Geometry: final body of the model. Coordinates: model frame, mm. A direction names the side the tool comes from. Coordinates: 2 decimals unless noted, no trailing zeros. Loops run counter-clockwise (first coordinate to the right, second up) from the corner with the lowest first, then second, coordinate; pieces in that order, holes last. Notation, with made-up numbers: (-28, 78.25) - (-2, 78.25) arc R11 cw to (-2, 85.25) - close; hole circle Ø5 at (69.25, -40). An arc over 180 degrees is marked (long way). Answer in a Markdown table with one row per item.
from build123d import *

# Parameters (mm, degrees)
SKETCH_1_R               = 23.5
EXTRUDE_1_DEPTH          = 4
SKETCH_2_R               = 5.85
EXTRUDE_2_DEPTH          = 7
SKETCH_3_R               = 2.5
CUT_EXTRUDE_1_DEPTH      = 3.4
SKETCH_4_R               = 2.1
CUT_EXTRUDE_2_DEPTH      = 5
PATTERN_CIRCULAR_1_COUNT = 4
SKETCH_5_R               = 2
CUT_EXTRUDE_3_DEPTH      = 8.6


with BuildPart() as part:
    # 草圖1 → 填料-伸長1 (new body)
    with BuildSketch(Plane(origin=(0, 0, 0), x_dir=(1, 0, 0), z_dir=(0, 1, 0))):
        Circle(SKETCH_1_R)
    extrude(amount=EXTRUDE_1_DEPTH)

    # 草圖2 → 填料-伸長2 (add)
    with BuildSketch(Plane(origin=(0, 4, 0), x_dir=(1, 0, 0), z_dir=(0, 1, 0))):
        Circle(SKETCH_2_R)
    extrude(amount=EXTRUDE_2_DEPTH)

    # 草圖3 → 除料-伸長1 (cut)
    with BuildSketch(Plane(origin=(0, 11, 0), x_dir=(1, 0, 0), z_dir=(0, 1, 0))):
        Circle(SKETCH_3_R)
    extrude(amount=-CUT_EXTRUDE_1_DEPTH, mode=Mode.SUBTRACT)

    # 草圖4 → 除料-伸長2 (cut, through all)
    with BuildSketch(Plane(origin=(0, 4, 0), x_dir=(1, 0, 0), z_dir=(0, 1, 0))):
        with Locations((-15.5, 0)):
            Circle(SKETCH_4_R)
        with Locations((-15.5, 8.5)):
            Circle(SKETCH_4_R)
        with Locations((-15.5, -8.5)):
            Circle(SKETCH_4_R)
    cut_extrude_2 = extrude(amount=-CUT_EXTRUDE_2_DEPTH, mode=Mode.SUBTRACT)

    # 環狀複製排列1: 除料-伸長2 ×4 about axis
    pattern_circular_1_axis = Axis((0, 0, 0), (0, 1, 0))
    for i in range(1, PATTERN_CIRCULAR_1_COUNT):
        add(cut_extrude_2.rotate(pattern_circular_1_axis, i * 360 / PATTERN_CIRCULAR_1_COUNT), mode=Mode.SUBTRACT)

    # 草圖5 → 除料-伸長3 (cut, through all)
    with BuildSketch(Plane(origin=(0, 7.6, 0), x_dir=(1, 0, 0), z_dir=(0, 1, 0))):
        Circle(SKETCH_5_R)
    extrude(amount=-CUT_EXTRUDE_3_DEPTH, mode=Mode.SUBTRACT)


solid = part.part
(1) First-contact query: pin 1 Ø5 at (x, z) = (-7.5, 10.5) entering from -Y; pin 2 Ø2 at (x, y) = (-1, 7.5) entering from +Z; pin 3 Ø5.5 at (x, z) = (-15.5, 0) entering from +Y; pin 4 Ø2.5 at (x, z) = (-1, -0.5) entering from +Y. Flat tips, straight axial feed; report the tip coordinate or a pass-through.
Verdict:
| item | result |
|---|---|
| pin 1 | stops at y = 0 |
| pin 2 | stops at z = 5.85 |
| pin 3 | stops at y = 4 |
| pin 4 | stops at y = 7.6 |
(2) Cut plane A-A on y = 1.75. State how many separate pieces and enclosed holes the cut face has, then the cut area to 3 significant figures.
Verdict:
| item | result |
|---|---|
| separate pieces | 1 |
| enclosed holes | 13 |
| area | 1,560 mm² |
(3) Cut plane B-B on z = -7. Output: boundary loops of the cut face in (x, y).
Verdict:
| item | result |
|---|---|
| outline | (-22.43, 0) - (-16.97, 0) - (-16.97, 4) - (-22.43, 4) - close; (-14.03, 0) - (14.03, 0) - (14.03, 4) - (-14.03, 4) - close; (16.97, 0) - (22.43, 0) - (22.43, 4) - (16.97, 4) - close |
(4) Access query for faces 4 (the face through (-1, 7.6, -2)), 5 (the face through (0, 0, 5)). Directions: +Z, -Z, +X, -X, +Y, -Y. A direction counts if a zero-diameter tool reaches every point of the face in a straight line with its end or side. Return the directions, or none.
Verdict:
| item | result |
|---|---|
| face 4 | +Y |
| face 5 | +Z, -Z, +X, -X, -Y |
(5) Ray query, probe 1 along X at (y, z) = (3.25, -15.5); probe 2 along Z at (x, y) = (0, 5.5); probe 3 along Z at (x, y) = (0, 9.55). Return the intervals inside material, ascending.
Verdict:
| item | result |
|---|---|
| probe 1 | x = -17.66 to -10.6, -6.4 to -2.1, 2.1 to 6.4, 10.6 to 17.66 |
| probe 2 | z = -5.85 to -2, 2 to 5.85 |
| probe 3 | z = -5.85 to -2.5, 2.5 to 5.85 |
(6) Cut plane D-D on z = 0. Output: boundary loops of the cut face in (x, y), then the cut area to 3 significant figures.
Verdict:
| item | result |
|---|---|
| outline | (-23.5, 0) - (-17.6, 0) - (-17.6, 4) - (-23.5, 4) - close; (-13.4, 0) - (-2, 0) - (-2, 7.6) - (-2.5, 7.6) - (-2.5, 11) - (-5.85, 11) - (-5.85, 4) - (-13.4, 4) - close; (2, 0) - (13.4, 0) - (13.4, 4) - (5.85, 4) - (5.85, 11) - (2.5, 11) - (2.5, 7.6) - (2, 7.6) - close; (17.6, 0) - (23.5, 0) - (23.5, 4) - (17.6, 4) - close |
| area | 189 mm² |
(7) Cut plane C-C on x = 10. Output: boundary loops of the cut face in (y, z).
Verdict:
| item | result |
|---|---|
| outline | (0, -21.27) - (4, -21.27) - (4, -16.97) - (0, -16.97) - close; (0, -14.03) - (4, -14.03) - (4, 14.03) - (0, 14.03) - close; (0, 16.97) - (4, 16.97) - (4, 21.27) - (0, 21.27) - close |
(8) Pull-direction query (X, two-part tool) for faces 1 (the face through (0, 11, 3)), 2 (the face through (22.4, 2, -7.1)), 3 (the face through (-0.54, 9.32, 2.44)); classes: pulls with the +X half, pulls with the -X half, needs draft (parallel to the pull), parting line crosses it, or undercut.
Verdict:
| item | result |
|---|---|
| face 1 | needs draft |
| face 2 | parting line crosses it |
| face 3 | undercut |
